```python
from build123d import *

# Parameters (mm, degrees)
SKETCH002_R  = 150
PAD002_DEPTH = 185
PAD003_DEPTH = 105
PAD004_DEPTH = 70


with BuildPart() as part:
    # Sketch002 → Pad002 (new body)
    with BuildSketch(Plane.YZ):
        Circle(SKETCH002_R)
    extrude(amount=PAD002_DEPTH)

    # Sketch003 (on Face3 of Pad002) → Pad003 (join)
    with BuildSketch(Plane.YZ.offset(185)):
        with BuildLine():
            Line((-3, 14.696938), (-3, 12.196938))
            Line((-3, 12.196938), (3, 12.196938))
            Line((3, 12.196938), (3, 14.696938))
            ThreePointArc((-3, 14.696938), (0, -15), (3, 14.696938))
        make_face()
    extrude(amount=PAD003_DEPTH)

    # Sketch004 (on Face2 of Pad003) → Pad004 (join)
    with BuildSketch(Plane(origin=(0, 0, 0), x_dir=(0, 1, 0), z_dir=(-1, 0, 0))):
        with BuildLine():
            Line((-3, -14.696938), (-3, -12.196938))
            Line((-3, -12.196938), (3, -12.196938))
            Line((3, -12.196938), (3, -14.696938))
            ThreePointArc((3, -14.696938), (0, 15), (-3, -14.696938))
        make_face()
    extrude(amount=PAD004_DEPTH)


with BuildPart() as part_1:
    # Body001 placement: moved
    add(part.part.moved(Location((-110, 174, 189))))


solid = part_1.part
```
Input: part model. Units: mm. Frame: model coordinates. A direction names the side the tool comes from. Coordinates: 2 decimals unless noted, no trailing zeros. Write each loop counter-clockwise with the first axis right and the second up, starting at its lowest first coordinate (ties: lowest second). Pieces come first, ordered by that corner, then holes. Notation, with made-up numbers: (80.5, -1) -> (93.5, -1) arc R16 cw to (93.5, 24) -> close; hole circle Ø1 at (32.5, 51). An arc over 180 degrees is marked (long way). Answer as a JSON object with one key per item and string values.
1. Section C-C on y = 102. Return the cut outline in (x, z), then the cut area to 3 significant figures.
Result set:
{"outline": "(-110, 57.41) -> (75, 57.41) -> (75, 320.59) -> (-110, 320.59) -> close", "area": "48,700 mm2"}
2. First-contact query: P1, Ø5, axis at x = -133, y = 174, coming from the +Z side; P2, Ø1.2, axis at x = 138.5, z = 203, coming from the +Y side; P3, Ø12, axis at y = 150, z = 112.5, coming from the +X side. Flat tips, straight axial feed; report the tip coordinate or a pass-through.
Result set:
{"P1": "stops at z = 201.2", "P2": "stops at y = 180.74", "P3": "stops at x = 75"}
3. Section B-B on x = 109.5. Return the cut outline in (y, z).
Result set:
{"outline": "(171, 201.2) -> (171, 203.7) arc R15 ccw (long way) to (177, 203.7) -> (177, 201.2) -> close"}
4. Access query for faces 3 (the face through (-18.795, 54.965, 97.727)), 4 (the face through (126.765, 173.383, 174.013)). Directions: +Z, -Z, +X, -X, +Y, -Y. A direction counts if a zero-diameter tool reaches every point of the face in a straight line with its end or side. Return the directions, or none.
Result set:
{"face 3": "+X, -X", "face 4": "+X"}
5. Mould query, pull axis Y, two halves, no side actions, for faces 1 (the face through (-180, 174, 189)), 2 (the face through (-144.51, 174.617, 174.013)). Classes: released by +Y, released by -Y, zero draft, split by the parting line, or undercut.
Result set:
{"face 1": "zero draft", "face 2": "split by the parting line"}
6. Section D-D on x = -61. Return the cut outline in (y, z).
Result set:
{"outline": "circle Ø300 at (174, 189)"}
7. Section A-A on z = 189. Return the cut outline in (x, y).
Result set:
{"outline": "(-180, 159) -> (-110, 159) -> (-110, 24) -> (75, 24) -> (75, 159) -> (180, 159) -> (180, 189) -> (75, 189) -> (75, 324) -> (-110, 324) -> (-110, 189) -> (-180, 189) -> close"}
8. Material intervals for line 1 (X direction, y = 270.5, z = 262); line 2 (Y direction, x = 70, z = 134); line 3 (Z direction, x = -108.5, y = 217), sorted ascending. Write a range as from..to.
Result set:
{"line 1": "x = -110..75", "line 2": "y = 34.45..313.55", "line 3": "z = 45.3..332.7"}
